Build history of the part. All positions in model axes, mm. Face numbers are marked on the shaded views. A direction names the side the tool comes from. Coordinates: 2 decimals unless noted, no trailing zeros. Write each loop counter-clockwise with the first axis right and the second up, starting at its lowest first coordinate (ties: lowest second). Pieces come first, ordered by that corner, then holes. Notation, with made-up numbers: (75.25, -19.75) -> (91.25, -19.75) arc R22 cw to (91.25, -12.75) -> close; hole circle Ø3 at (-21.75, -12.5). An arc over 180 degrees is marked (long way). Write each question's results on one line, items separated by ' | '. Start each with the question number.
Q1. Drill centre lines: line 1 (Y direction, x = 3.4, z = -11.5); line 2 (Y direction, x = 0.6, z = -6.5); line 3 (Z direction, x = 0.6, y = -4). Where is each one in solid material? Low to high.
Q2. Saw through at C-C on y = -4. Give the cut face in (x, z).
Q3. Saw through at B-B on x = 2.4. Give the cut face in (y, z).
Q4. Tool access for the marked faces 1, 2 and 3: list every direction of +Z, -Z, +X, -X, +Y, -Y with a clear straight run to the whole face (end or side of a thin tool).
Q5. Drop flat-ended pins along their axis: pin 1 Ø2 at (x, y) = (2, 25) entering from +Z; pin 2 Ø2 at (x, z) = (2, 12.5) entering from +Y. Give the stop position or say it passes through.
Q6. Saw through at D-D on z = 19.5. Give the cut face in (x, y).
Q7. Saw through at A-A on y = 20.5. Give the cut face in (x, z), and give its area (3 significant figures).
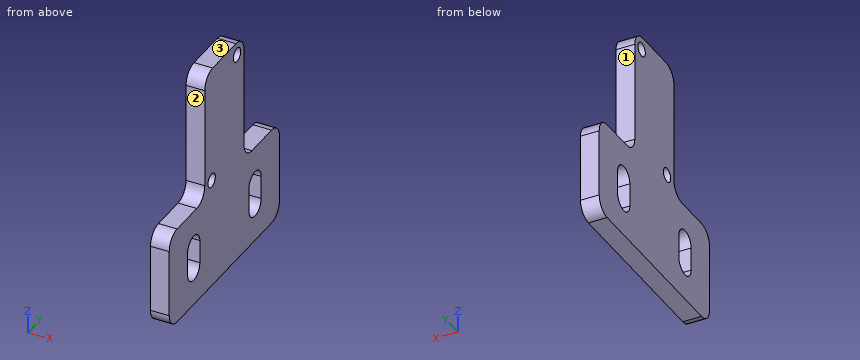
from build123d import *

# Parameters (mm, degrees)
SKETCH1_W           = 16
SKETCH1_H           = 28
SKETCH1_R           = 1.5
SKETCH1_W_2         = 45
SKETCH1_H_2         = 21
BOSS_EXTRUDE1_DEPTH = 4
FILLET1_R           = 3.25


with BuildPart() as part:
    # Sketch1 → Boss-Extrude1 (new body)
    # profile 1 of 2: a face of its own
    with BuildSketch(Plane.YZ):
        with Locations((8, 14)):
            Rectangle(SKETCH1_W, SKETCH1_H)
        with Locations(Location((13.187246979, 25.187246979, 0), (0, 0, 270))):
            Circle(SKETCH1_R, mode=Mode.SUBTRACT)
        with Locations(Location((2.812753021, 2.812753021, 0), (0, 0, 270))):
            Circle(SKETCH1_R, mode=Mode.SUBTRACT)
    # profile 2 of 2: a face of its own
    with BuildSketch(Plane.YZ):
        with Locations((8, -10.5)):
            Rectangle(SKETCH1_W_2, SKETCH1_H_2)
        with BuildLine():
            Line((-2, -8), (-2, -13))
            ThreePointArc((-2, -13), (-4.5, -15.5), (-7, -13))
            Line((-7, -13), (-7, -8))
            ThreePointArc((-7, -8), (-4.5, -5.5), (-2, -8))
        make_face(mode=Mode.SUBTRACT)
        with BuildLine():
            Line((23, -8), (23, -13))
            ThreePointArc((23, -13), (20.5, -15.5), (18, -13))
            Line((18, -13), (18, -8))
            ThreePointArc((18, -8), (20.5, -5.5), (23, -8))
        make_face(mode=Mode.SUBTRACT)
    extrude(amount=BOSS_EXTRUDE1_DEPTH)

    # Fillet1
    fillet1_edges = [part.edges().sort_by_distance(p)[0] for p in [
        (2, 0, 28),
        (2, 16, 28),
        (2, 16, 0),
        (2, 30.5, 0),
        (2, 30.5, -21),
        (2, -14.5, -21),
        (2, -14.5, 0),
        (2, 0, 0),
    ]]
    fillet(fillet1_edges, radius=FILLET1_R)


solid = part.part
Returned:
1) line 1: y = -14.5 to -7, -2 to 18, 23 to 30.5 | line 2: y = -14.5 to -6.5, -2.5 to 18.5, 22.5 to 30.5 | line 3: z = -21 to -15.45, -5.55 to 0
2) outline: (0, -21) -> (4, -21) -> (4, -15.45) -> (0, -15.45) -> close; (0, -5.55) -> (4, -5.55) -> (4, 0) -> (0, 0) -> close
3) outline: (-14.5, -17.75) arc R3.25 ccw to (-11.25, -21) -> (27.25, -21) arc R3.25 ccw to (30.5, -17.75) -> (30.5, -3.25) arc R3.25 ccw to (27.25, 0) -> (19.25, 0) arc R3.25 cw to (16, 3.25) -> (16, 24.75) arc R3.25 ccw to (12.75, 28) -> (3.25, 28) arc R3.25 ccw to (0, 24.75) -> (0, 3.25) arc R3.25 cw to (-3.25, 0) -> (-11.25, 0) arc R3.25 ccw to (-14.5, -3.25) -> close; hole (-7, -13) arc R2.5 ccw to (-2, -13) -> (-2, -8) arc R2.5 ccw to (-7, -8) -> close; hole circle Ø3 at (2.81, 2.81); hole circle Ø3 at (13.19, 25.19); hole (18, -13) arc R2.5 ccw to (23, -13) -> (23, -8) arc R2.5 ccw to (18, -8) -> close
4) face 1: +Z, +X, -X, +Y | face 2: +Z, +X, -X, -Y | face 3: +Z, +X, -X, +Y, -Y
5) pin 1: stops at z = 0 | pin 2: stops at y = 16
6) outline: (0, 0) -> (4, 0) -> (4, 16) -> (0, 16) -> close
7) outline: (0, -21) -> (4, -21) -> (4, -15.5) -> (0, -15.5) -> close; (0, -5.5) -> (4, -5.5) -> (4, 0) -> (0, 0) -> close | area: 44.0 mm2
